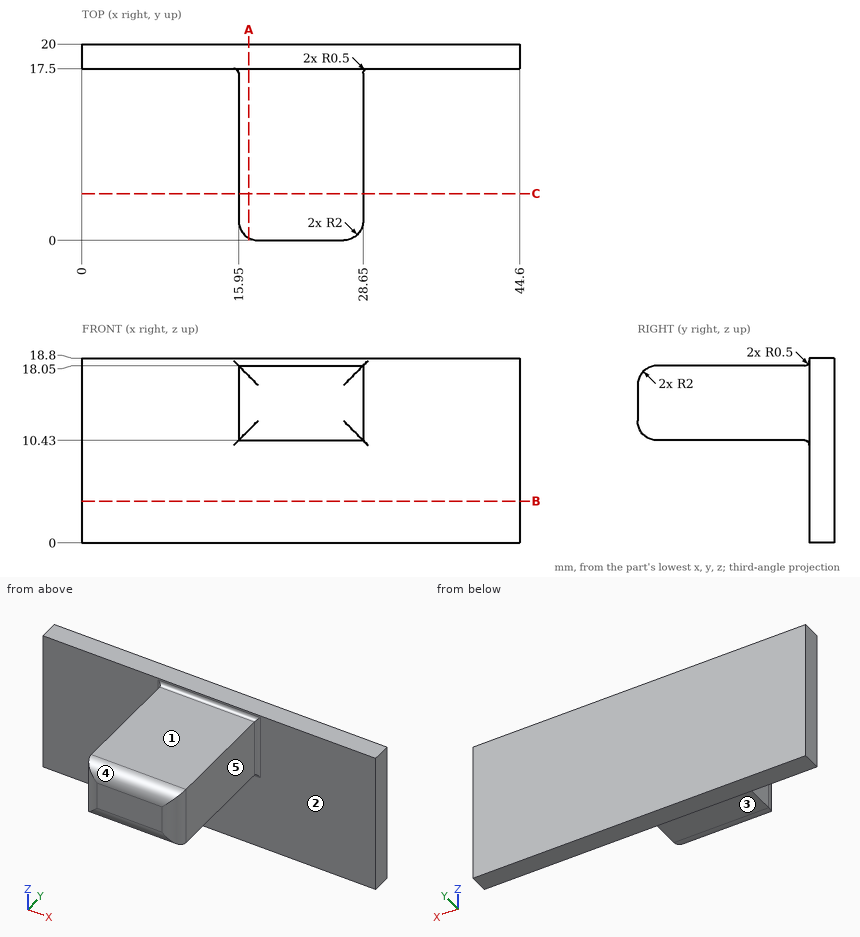
The drawing under review shows one solid part. Ordinate dimensions are in mm from its lowest x, y, z. A direction names the side the tool comes from. Give positions to 0.01 mm unless a question says otherwise; leave off trailing zeros. Write each loop counter-clockwise with the first axis right and the second up, starting at its lowest first coordinate (ties: lowest second). Pieces come first, ordered by that corner, then holes. Notation, with made-up numbers: (42, -7) -> (101, -7) arc R13 ccw to (101, 7) -> close; hole circle Ø6 at (40, -32). An arc over 180 degrees is marked (long way). Answer in a Markdown table with one row per item.
(1) For the marked faces 4 and 5, list the 3-axis set-ups (+Z, -Z, +X, -X, +Y, -Y) from which the entire face can be reached by the end or side of a thin tool; tool diameter is ignored.
Results:
| item | result |
|---|---|
| face 4 | +Z, +X, -X, -Y |
| face 5 | +Z, -Z, +X, -Y |
(2) Clearance check with flat-ended pins moving along their axes: pin 1 (1.5 mm diameter, centred on x = 10.5, z = 4.5, fed in from -Y); pin 2 (6.5 mm diameter, centred on x = 23, y = 9.5, fed in from -Z); pin 3 (4 mm diameter, centred on x = 21, y = 13, fed in from +Z); pin 4 (3 mm diameter, centred on y = 10, z = 7, fed in from +X). State where each tip first meets the part, or that it passes through.
Results:
| item | result |
|---|---|
| pin 1 | y = 17.5 |
| pin 2 | z = 10.43 |
| pin 3 | z = 18.05 |
| pin 4 | through |
(3) Consider section A-A (x = 17). State the section outline as (y, z) points.
Results:
| item | result |
|---|---|
| outline | (0.24, 11.48) arc R2 ccw to (2, 10.43) -> (17, 10.43) arc R0.5 cw to (17.5, 9.93) -> (17.5, 0) -> (20, 0) -> (20, 18.8) -> (17.5, 18.8) -> (17.5, 18.55) arc R0.5 cw to (17, 18.05) -> (2, 18.05) arc R2 ccw to (0.24, 17) -> close |
(4) Mouldability with a two-part tool opening along Z and no side actions: class the marked faces 1, 2 and 3 as +Z half, -Z half, draft (parallel to the pull), parting line (faces both ways), or undercut.
Results:
| item | result |
|---|---|
| face 1 | +Z half |
| face 2 | draft |
| face 3 | -Z half |
(5) To check wall thickness, follow probe 1 along Y at (x, z) = (19, 8); probe 2 along X at (y, z) = (8, 15); probe 3 along Z at (x, y) = (16, 3). State the ranges of each line that lie inside material, in increasing order.
Results:
| item | result |
|---|---|
| probe 1 | 17.5 to 20 |
| probe 2 | 15.95 to 28.65 |
| probe 3 | 10.43 to 18.05 |
(6) Consider section B-B (z = 4.25). State the section outline as (x, y) points, then the cut area to 4 significant figures.
Results:
| item | result |
|---|---|
| outline | (0, 17.5) -> (44.6, 17.5) -> (44.6, 20) -> (0, 20) -> close |
| area | 111.5 mm2 |
(7) Consider section C-C (y = 4.75). State the section outline as (x, z) points, then the cut area to 3 significant figures.
Results:
| item | result |
|---|---|
| outline | (15.95, 10.43) -> (28.65, 10.43) -> (28.65, 18.05) -> (15.95, 18.05) -> close |
| area | 96.8 mm2 |
